Verification items for the finished model (mm, model axes). Coordinates: 2 decimals unless noted, no trailing zeros. Write each loop counter-clockwise with the first axis right and the second up, starting at its lowest first coordinate (ties: lowest second). Pieces come first, ordered by that corner, then holes. Notation, with made-up numbers: (87, 34.5) - (119, 34.5) arc R30 cw to (119, 56.5) - close; hole circle Ø11 at (85, 48.5). An arc over 180 degrees is marked (long way). Use CSV: the item, a comma, the result in double quotes. Start each with the question number.
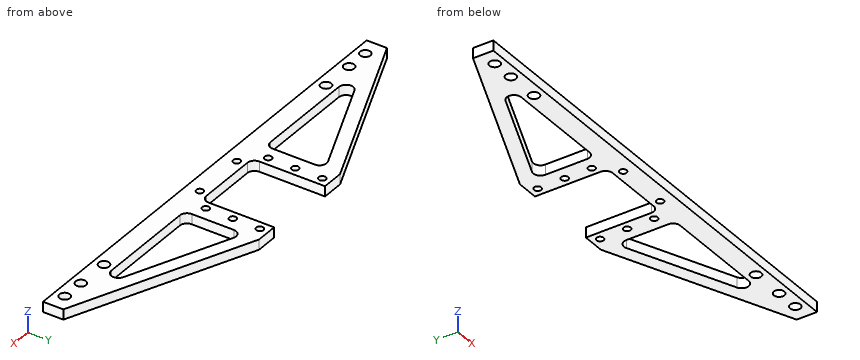
```python
from build123d import *

# Parameters (mm, degrees)
SKETCH_1_R          = 1.05
SKETCH_1_R_2        = 1.55
EXTRUDE_1_DEPTH     = 3
SKETCH_2_R          = 1.55
CUT_EXTRUDE_1_DEPTH = 3


with BuildPart() as part:
    # ｽｹｯﾁ1 → ﾎﾞｽ - 押し出し1 (new body)
    with BuildSketch(Plane.XY):
        with BuildLine():
            Line((-11, 4.6), (-11, 24))
            Line((-11, 24), (-17.5, 24))
            Line((-17.5, 24), (-70, 2))
            Line((-70, 2), (-70, -4))
            Line((-70, -4), (-17.5, -4))
            Line((-17.5, -4), (17.5, -4))
            Line((17.5, -4), (70, -4))
            Line((70, -4), (70, 2))
            Line((70, 2), (17.5, 24))
            Line((17.5, 24), (11, 24))
            Line((11, 24), (11, 4.6))
            ThreePointArc((11, 4.6), (10.38492424, 3.11507576), (8.9, 2.5))
            Line((8.9, 2.5), (-8.9, 2.5))
            ThreePointArc((-8.9, 2.5), (-10.38492424, 3.11507576), (-11, 4.6))
        make_face()
        with Locations((-13.5, 5.5)):
            Circle(SKETCH_1_R, mode=Mode.SUBTRACT)
        with Locations((-8, 0)):
            Circle(SKETCH_1_R, mode=Mode.SUBTRACT)
        with Locations((8, 0)):
            Circle(SKETCH_1_R, mode=Mode.SUBTRACT)
        with Locations((-13.5, 13.5)):
            Circle(SKETCH_1_R, mode=Mode.SUBTRACT)
        with Locations((-13.5, 21.5)):
            Circle(SKETCH_1_R, mode=Mode.SUBTRACT)
        with Locations((13.5, 21.5)):
            Circle(SKETCH_1_R, mode=Mode.SUBTRACT)
        with Locations((13.5, 13.5)):
            Circle(SKETCH_1_R, mode=Mode.SUBTRACT)
        with Locations((13.5, 5.5)):
            Circle(SKETCH_1_R, mode=Mode.SUBTRACT)
        with Locations((-65, -1)):
            Circle(SKETCH_1_R_2, mode=Mode.SUBTRACT)
        with Locations(Location((65, -1, 0), (0, 0, 180))):
            Circle(SKETCH_1_R_2, mode=Mode.SUBTRACT)
        with BuildLine():
            Line((-17.5, 4.1), (-17.5, 16.506066998))
            ThreePointArc((-17.5, 16.506066998), (-18.436901101, 18.254552329), (-20.411619954, 18.442887344))
            Line((-20.411619954, 18.442887344), (-50.017007109, 6.036820345))
            ThreePointArc((-50.017007109, 6.036820345), (-51.264188108, 3.686069284), (-49.205387155, 2))
            Line((-49.205387155, 2), (-19.6, 2))
            ThreePointArc((-19.6, 2), (-18.11507576, 2.61507576), (-17.5, 4.1))
        make_face(mode=Mode.SUBTRACT)
        with BuildLine():
            Line((20.411619954, 18.442887344), (50.017007109, 6.036820345))
            ThreePointArc((50.017007109, 6.036820345), (51.264188108, 3.686069284), (49.205387155, 2))
            Line((49.205387155, 2), (19.6, 2))
            ThreePointArc((19.6, 2), (18.11507576, 2.61507576), (17.5, 4.1))
            Line((17.5, 4.1), (17.5, 16.506066998))
            ThreePointArc((17.5, 16.506066998), (18.436901101, 18.254552329), (20.411619954, 18.442887344))
        make_face(mode=Mode.SUBTRACT)
    extrude(amount=EXTRUDE_1_DEPTH)

    # ｽｹｯﾁ2 → ｶｯﾄ - 押し出し1 (cut)
    with BuildSketch(Plane.XY.offset(3)):
        with Locations((-48, -1)):
            Circle(SKETCH_2_R)
        with Locations(Location((48, -1, 0), (0, 0, 180))):
            Circle(SKETCH_2_R)
        with Locations((-58, -1)):
            Circle(SKETCH_2_R)
        with Locations(Location((58, -1, 0), (0, 0, 180))):
            Circle(SKETCH_2_R)
    extrude(amount=-CUT_EXTRUDE_1_DEPTH, mode=Mode.SUBTRACT)


solid = part.part
```
Q1. Scan lines: line 1 along Y through (x, z) = (-13.5, 1.55); line 2 along X through (y, z) = (3.25, 0.5); line 3 along X through (y, z) = (11.5, 2.25). Record each from-to range of solid material in increasing order. Write a range as from..to.
Q2. Cross-section at A-A (x = 58). Record the cut outline in (y, z).
Q3. Cross-section at B-B (z = 2). State how many separate pieces and enclosed holes the cut face has, plus the area to 3 significant figures.
Q4. Gauge pin test, flat ends, axial feed: pin 1 (0.9 mm diameter, centred on y = 11, z = 1, fed in from -X); pin 2 (1 mm diameter, centred on x = 8, z = 1.5, fed in from +Y); pin 3 (1.5 mm diameter, centred on y = 10, z = 2, fed in from +X); pin 4 (3.5 mm diameter, centred on x = 48, y = -1, fed in from -Z). Record the tip position at first contact, or that the pin passes through.
Reply:
1,line 1,"-4..4.45, 6.55..12.45, 14.55..20.45, 22.55..24"
1,line 2,"-67.02..-51.13, -17.68..-10.51, 10.51..17.68, 51.13..67.02"
1,line 3,"-47.33..-36.98, -17.5..-11, 11..17.5, 36.98..47.33"
2,outline,"(-4, 0) - (-2.55, 0) - (-2.55, 3) - (-4, 3) - close; (0.55, 0) - (7.03, 0) - (7.03, 3) - (0.55, 3) - close"
3,separate pieces,"1"
3,enclosed holes,"16"
3,area,"1,510 mm^2"
4,pin 1,"x = -49.6"
4,pin 2,"y = 2.5"
4,pin 3,"x = 52.7"
4,pin 4,"z = 0"
